Source: CAD feature listing. Evaluate the final solid. Frame: model axes, mm. Coordinates: 2 decimals unless noted, no trailing zeros. Loops run counter-clockwise (first coordinate to the right, second up) from the corner with the lowest first, then second, coordinate; pieces in that order, holes last.
Item 1: Section query D-D, the plane z = -90. Return the cut outline in (x, y).
Item 2: Section query A-A, the plane z = -60. Return the cut outline in (x, y).
Item 3: Section query B-B, the plane x = -64.5. Return the cut outline in (y, z).
Item 4: Pin query (flat end, axial travel): pin 1 Ø2.5 at (x, y) = (-147.5, 3.5) entering from +Z. Return the tip coordinate at first contact, or that it passes through.
Item 5: Section query C-C, the plane y = 2.95. Return the cut outline in (x, z), then the cut area to 3 significant figures.
Item 6: Line query: probe 1 along X at (y, z) = (3.9, -60); probe 2 along X at (y, z) = (4.1, -67.5); probe 3 along Z at (x, y) = (-68, 0.8). Output: solid intervals per line, ascending.
```python
from build123d import *

# Parameters (mm, degrees)
SKETCH1_W           = 300
SKETCH1_H           = 120
BOSS_EXTRUDE1_DEPTH = 5
SKETCH2_R           = 45
SKETCH2_W           = 60
SKETCH2_H           = 5
CUT_EXTRUDE1_DEPTH  = 5


with BuildPart() as part:
    # Sketch1 → Boss-Extrude1 (new body)
    with BuildSketch(Plane(origin=(0, 0, 0), x_dir=(1, 0, 0), z_dir=(0, 1, 0))):
        with Locations((-150, 60)):
            Rectangle(SKETCH1_W, SKETCH1_H)
    extrude(amount=BOSS_EXTRUDE1_DEPTH)

    # Sketch2 → Cut-Extrude1 (cut)
    with BuildSketch(Plane(origin=(0, 5, 0), x_dir=(1, 0, 0), z_dir=(0, 1, 0))):
        with Locations(Location((-64.5, 60, 0), (0, 0, 270))):
            Circle(SKETCH2_R)
        with Locations(Location((-235.5, 60, 0), (0, 0, 270))):
            Circle(SKETCH2_R)
        with Locations((-150, 2.5)):
            Rectangle(SKETCH2_W, SKETCH2_H)
    extrude(amount=-CUT_EXTRUDE1_DEPTH, mode=Mode.SUBTRACT)


solid = part.part
```
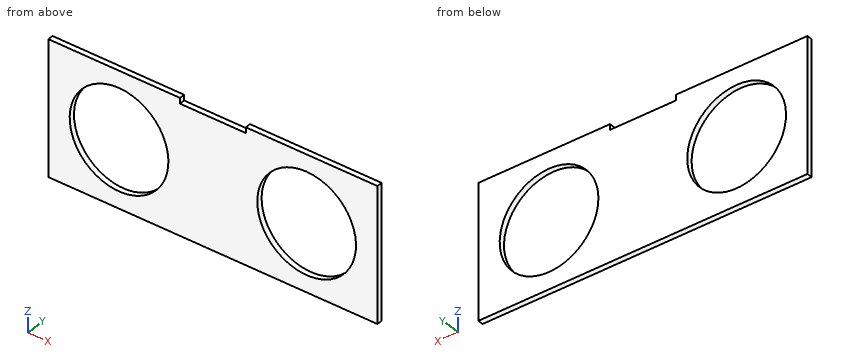
Verdict:
1. outline: (-300, 0) - (-269.04, 0) - (-269.04, 5) - (-300, 5) - close; (-201.96, 0) - (-98.04, 0) - (-98.04, 5) - (-201.96, 5) - close; (-30.96, 0) - (0, 0) - (0, 5) - (-30.96, 5) - close
2. outline: (-300, 0) - (-280.5, 0) - (-280.5, 5) - (-300, 5) - close; (-190.5, 0) - (-109.5, 0) - (-109.5, 5) - (-190.5, 5) - close; (-19.5, 0) - (0, 0) - (0, 5) - (-19.5, 5) - close
3. outline: (0, -120) - (5, -120) - (5, -105) - (0, -105) - close; (0, -15) - (5, -15) - (5, 0) - (0, 0) - close
4. pin 1: stops at z = -5
5. outline: (-300, -120) - (0, -120) - (0, 0) - (-120, 0) - (-120, -5) - (-180, -5) - (-180, 0) - (-300, 0) - close; hole circle Ø90 at (-235.5, -60); hole circle Ø90 at (-64.5, -60)
5. area: 23,000 mm2
6. probe 1: x = -300 to -280.5, -190.5 to -109.5, -19.5 to 0
6. probe 2: x = -300 to -279.87, -191.13 to -108.87, -20.13 to 0
6. probe 3: z = -120 to -104.86, -15.14 to 0
